The figure shows three views and two pictorial views of one solid part (mm, origin at its lowest corner). Answer the questions. A direction names the side the tool comes from. Give positions to 0.01 mm unless a question says otherwise; leave off trailing zeros. Write each loop counter-clockwise with the first axis right and the second up, starting at its lowest first coordinate (ties: lowest second). Pieces come first, ordered by that corner, then holes. Notation, with made-up numbers: (-28, 8) -> (17, 8) arc R26 cw to (17, 40) -> close; hole circle Ø7 at (61.5, 35). An arc over 180 degrees is marked (long way). Use a Markdown table: item, result.
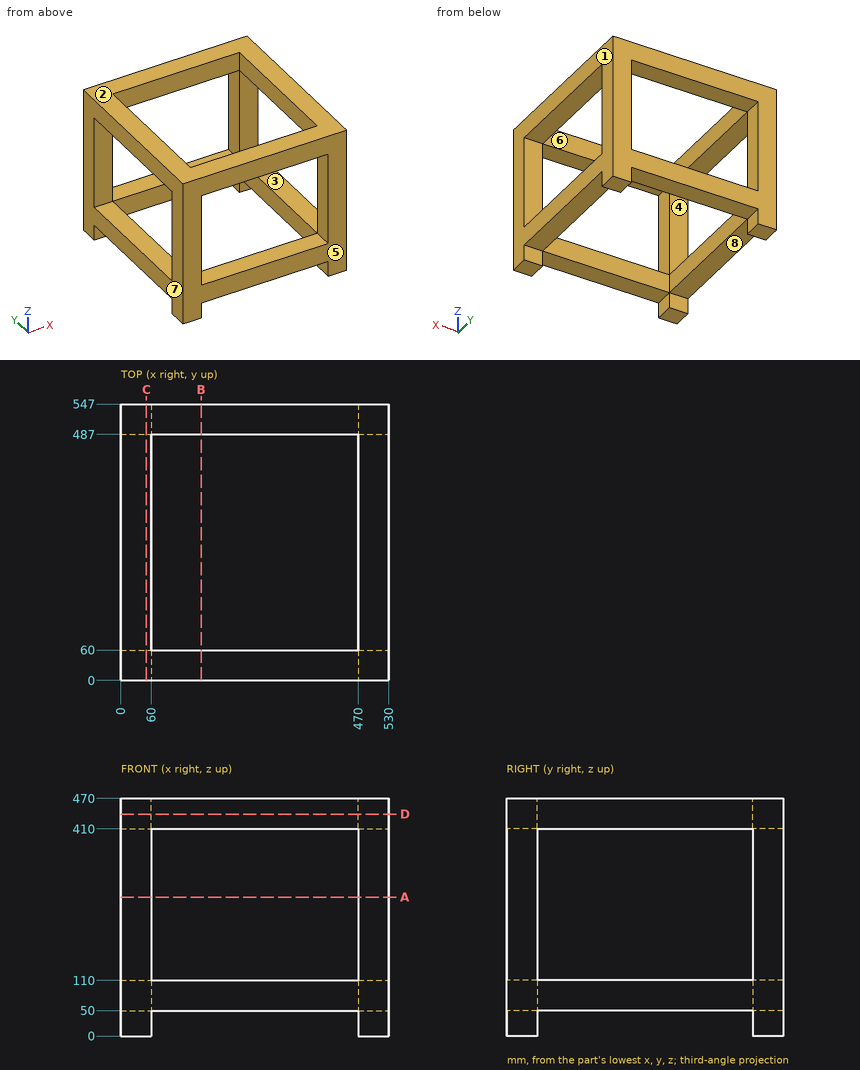
Item 1: A cutting plane is placed at D-D (z = 439). Give the vertices of the cut face in (x, y).
Return value:
| item | result |
|---|---|
| outline | (0, 0) -> (530, 0) -> (530, 547) -> (0, 547) -> close; hole (60, 60) -> (470, 60) -> (470, 487) -> (60, 487) -> close |
Item 2: A tool of negligible diameter and unlimited length cuts with its end or side. For the marked faces 4, 5, 6, 7 and 8, from which of +Z, -Z, +X, -X, +Y, -Y can it reach the whole face along a straight path? Write none if from no direction.
Return value:
| item | result |
|---|---|
| face 4 | +X, -X |
| face 5 | +Z, -Z, +X, -X, -Y |
| face 6 | +Z, -Z |
| face 7 | +Z, -Z, -X, +Y, -Y |
| face 8 | -Z, +X, -X |
Item 3: For a pull along Z with two mould halves and no side action, classify the marked faces 1, 2 and 3 as +Z half, -Z half, draft (parallel to the pull), parting line (faces both ways), or undercut.
Return value:
| item | result |
|---|---|
| face 1 | draft |
| face 2 | +Z half |
| face 3 | undercut |
Item 4: A cutting plane is placed at B-B (x = 159). Give the vertices of the cut face in (y, z), then the cut area to 3 significant figures.
Return value:
| item | result |
|---|---|
| outline | (0, 50) -> (60, 50) -> (60, 110) -> (0, 110) -> close; (0, 410) -> (60, 410) -> (60, 470) -> (0, 470) -> close; (487, 50) -> (547, 50) -> (547, 110) -> (487, 110) -> close; (487, 410) -> (547, 410) -> (547, 470) -> (487, 470) -> close |
| area | 14,400 mm^2 |
Item 5: Straight lines are drawn through the part: line 1 along X through (y, z) = (290, 412.5); line 2 along Y through (x, z) = (480, 119.5); line 3 along Z through (x, y) = (420, 38.5). For each, find the intervals that lie inside material, in ascending order. Write a range as [from, to].
Return value:
| item | result |
|---|---|
| line 1 | [0, 60], [470, 530] |
| line 2 | [0, 60], [487, 547] |
| line 3 | [50, 110], [410, 470] |
Item 6: A cutting plane is placed at A-A (z = 275). Give the vertices of the cut face in (x, y), then the cut area to 3 significant figures.
Return value:
| item | result |
|---|---|
| outline | (0, 0) -> (60, 0) -> (60, 60) -> (0, 60) -> close; (0, 487) -> (60, 487) -> (60, 547) -> (0, 547) -> close; (470, 0) -> (530, 0) -> (530, 60) -> (470, 60) -> close; (470, 487) -> (530, 487) -> (530, 547) -> (470, 547) -> close |
| area | 14,400 mm^2 |
Item 7: A cutting plane is placed at C-C (x = 50.5). Give the vertices of the cut face in (y, z).
Return value:
| item | result |
|---|---|
| outline | (0, 0) -> (60, 0) -> (60, 50) -> (487, 50) -> (487, 0) -> (547, 0) -> (547, 470) -> (0, 470) -> close; hole (60, 110) -> (487, 110) -> (487, 410) -> (60, 410) -> close |
